Check sheet for the modelled part. Datum: model origin and axes. Units: mm. A direction names the side the tool comes from. Give positions to 0.01 mm unless a question says otherwise; leave off trailing zeros. Order: outer loops, then holes, each group sorted by start corner. A loop starts at its lowest first (then second) coordinate and runs counter-clockwise, first axis right, second up.
```python
from build123d import *

# Parameters (mm, degrees)
CROQUIS1_R              = 15
CROQUIS1_R_2            = 3
SALIENTE_EXTRUIR1_DEPTH = 25
CROQUIS2_R              = 16.5
CROQUIS2_R_2            = 3
SALIENTE_EXTRUIR2_DEPTH = 2
CROQUIS3_R              = 16.5
CROQUIS3_R_2            = 3
SALIENTE_EXTRUIR3_DEPTH = 2
CORTAR_EXTRUIR1_REACH   = 18.5
CROQUIS4_R              = 1.625
CROQUIS5_R              = 7.5
CORTAR_EXTRUIR2_DEPTH   = 16


with BuildPart() as part:
    # Croquis1 → Saliente-Extruir1 (new body)
    with BuildSketch(Plane(origin=(0, 0, 0), x_dir=(1, 0, 0), z_dir=(0, 1, 0))):
        Circle(CROQUIS1_R)
        Circle(CROQUIS1_R_2, mode=Mode.SUBTRACT)
    extrude(amount=SALIENTE_EXTRUIR1_DEPTH)

    # Croquis2 → Saliente-Extruir2 (add)
    with BuildSketch(Plane.XZ):
        Circle(CROQUIS2_R)
        Circle(CROQUIS2_R_2, mode=Mode.SUBTRACT)
    extrude(amount=-SALIENTE_EXTRUIR2_DEPTH)

    # Croquis3 → Saliente-Extruir3 (add)
    with BuildSketch(Plane(origin=(0, 25, 0), x_dir=(1, 0, 0), z_dir=(0, 1, 0))):
        Circle(CROQUIS3_R)
        Circle(CROQUIS3_R_2, mode=Mode.SUBTRACT)
    extrude(amount=-SALIENTE_EXTRUIR3_DEPTH)

    # Croquis4 → Cortar-Extruir1 (cut, up to next)
    with BuildSketch(Plane.XY, mode=Mode.PRIVATE) as cortar_extruir1_sk1:
        with Locations((0, 5)):
            Circle(CROQUIS4_R)
    cortar_extruir1_tool1 = extrude(cortar_extruir1_sk1.sketch, amount=-CORTAR_EXTRUIR1_REACH, mode=Mode.PRIVATE) & part.part
    add(cortar_extruir1_tool1.solids().sort_by_distance((0, 5, 0))[0], mode=Mode.SUBTRACT)

    # Croquis5 → Cortar-Extruir2 (cut)
    with BuildSketch(Plane(origin=(0, 25, 0), x_dir=(1, 0, 0), z_dir=(0, 1, 0))):
        Circle(CROQUIS5_R)
    extrude(amount=-CORTAR_EXTRUIR2_DEPTH, mode=Mode.SUBTRACT)


solid = part.part
```
Q1. Sectioned sample at B-B, the plane z = 0. Record the cut outline in (x, y), plus the area to 3 significant figures.
Q2. Draft check along X on faces 4 (the cylindrical face through (-14.985, 12.353, -0.66)), 5 (the cylindrical face through (-0.21, 6.61, -8.67)), 6 (the flat face through (-0.2, 0, -3.4)), 7 (the cylindrical face through (-0.65, 4.44, 2.93)). Enter one of: pulls with the +X half, pulls with the -X half, needs draft (parallel to the pull), parting line crosses it, or undercut.
Q3. Sectioned sample at D-D, the plane z = -10. Record the cut outline in (x, y) (3 decimals), plus the area to 3 significant figures.
Q4. Sectioned sample at A-A, the plane x = 0. Record the cut outline in (y, z) (3 decimals).
Q5. Sectioned sample at C-C, the plane y = 17.5. Record the cut outline in (x, z), plus the area to 3 significant figures.
Q6. Go/stop test with flat-tipped pins: P1, Ø4, axis at y = 3.5, z = 8.5, coming from the -X side; P2, Ø1, axis at x = -12.5, y = 14, coming from the +Z side; P3, Ø5, axis at y = 21.5, z = -10.5, coming from the +X side. Record where each tip stops, or that it passes through.
Q7. Material ranges on line 1 (Y direction, x = 0, z = -7.25) (3 decimals); line 2 (Z direction, x = 0, y = 2.25); line 3 (Z direction, x = 0, y = 17.5), recorded low to high.
Q8. Tool access check on faces 1 (the flat face through (4, 2, -15)), 2 (the flat face through (3.2, 9, -0.1)), 3 (the flat face through (3.4, 25, 7.1)). Record the directions out of +Z, -Z, +X, -X, +Y, -Y that give a thin tool (end or side, any length) a straight path to the whole face; none if there is none.
Filled in:
1. outline: (-16.5, 0) - (-3, 0) - (-3, 9) - (-7.5, 9) - (-7.5, 25) - (-16.5, 25) - (-16.5, 23) - (-15, 23) - (-15, 2) - (-16.5, 2) - close; (3, 0) - (16.5, 0) - (16.5, 2) - (15, 2) - (15, 23) - (16.5, 23) - (16.5, 25) - (7.5, 25) - (7.5, 9) - (3, 9) - close
1. area: 468 mm2
2. face 4: parting line crosses it
2. face 5: undercut
2. face 6: needs draft
2. face 7: undercut
3. outline: (-13.124, 0) - (13.124, 0) - (13.124, 2) - (11.18, 2) - (11.18, 23) - (13.124, 23) - (13.124, 25) - (-13.124, 25) - (-13.124, 23) - (-11.18, 23) - (-11.18, 2) - (-13.124, 2) - close; hole circle Ø3.25 at (0, 5)
3. area: 566 mm2
4. outline: (0, -16.5) - (2, -16.5) - (2, -15) - (3.375, -15) - (3.375, -3) - (0, -3) - close; (0, 3) - (9, 3) - (9, 7.5) - (25, 7.5) - (25, 16.5) - (23, 16.5) - (23, 15) - (2, 15) - (2, 16.5) - (0, 16.5) - close; (6.625, -15) - (23, -15) - (23, -16.5) - (25, -16.5) - (25, -7.5) - (9, -7.5) - (9, -3) - (6.625, -3) - close
5. outline: circle Ø30 at (0, 0); hole circle Ø15 at (0, 0)
5. area: 530 mm2
6. P1: stops at x = -14.86
6. P2: stops at z = 9
6. P3: stops at x = 14.14
7. line 1: y = 0 to 3.375, 6.625 to 9
7. line 2: z = -15 to -3, 3 to 15
7. line 3: z = -15 to -7.5, 7.5 to 15
8. face 1: none
8. face 2: +Y
8. face 3: +Z, -Z, +X, -X, +Y
